```python
from build123d import *

# Parameters (mm, degrees)
SKETCH_1_R      = 1.5
SKETCH_1_R_2    = 2.1
EXTRUDE_1_DEPTH = 90
FILLET_1_R      = 1


with BuildPart() as part:
    # 草图1 → 凸台-拉伸1 (new, symmetric)
    with BuildSketch(Plane.XY):
        Polygon((-10, 10), (-10, 4.8), (-8.34, 3.14), (-8.34, 5.4), (-5.753553391, 5.4), (-3.8, 3.446446609), (-3.8, -3.446446609), (-5.753553391, -5.4), (-8.34, -5.4), (-8.34, -3.14), (-10, -4.8), (-10, -10), (-4.8, -10), (-3.14, -8.34), (-5.4, -8.34), (-5.4, -5.753553391), (-3.446446609, -3.8), (3.446446609, -3.8), (5.4, -5.753553391), (5.4, -8.34), (3.14, -8.34), (4.8, -10), (10, -10), (10, -4.8), (8.34, -3.14), (8.34, -5.4), (5.753553391, -5.4), (3.8, -3.446446609), (3.8, 3.446446609), (5.753553391, 5.4), (8.34, 5.4), (8.34, 3.14), (10, 4.8), (10, 10), (4.8, 10), (3.14, 8.34), (5.4, 8.34), (5.4, 5.753553391), (3.446446609, 3.8), (-3.446446609, 3.8), (-5.4, 5.753553391), (-5.4, 8.34), (-3.14, 8.34), (-4.8, 10), align=None)
        with Locations(Location((-7.5, 7.5, 0), (0, 0, 180))):
            Circle(SKETCH_1_R, mode=Mode.SUBTRACT)
        with Locations(Location((0, 0, 0), (0, 0, 180))):
            Circle(SKETCH_1_R_2, mode=Mode.SUBTRACT)
        with Locations(Location((-7.5, -7.5, 0), (0, 0, 180))):
            Circle(SKETCH_1_R, mode=Mode.SUBTRACT)
        with Locations(Location((7.5, -7.5, 0), (0, 0, 180))):
            Circle(SKETCH_1_R, mode=Mode.SUBTRACT)
        with Locations(Location((7.5, 7.5, 0), (0, 0, 180))):
            Circle(SKETCH_1_R, mode=Mode.SUBTRACT)
    extrude(amount=EXTRUDE_1_DEPTH, both=True)

    # 圆角1
    fillet_1_edges = [part.edges().sort_by_distance(p)[0] for p in [
        (10, 10, 0),
        (10, -10, 0),
        (-10, -10, 0),
        (-10, 10, 0),
    ]]
    fillet(fillet_1_edges, radius=FILLET_1_R)


solid = part.part
```
Here's how the part is built. I have some questions about the finished solid (model axes, mm). Round coordinates to 2 decimals unless told otherwise and drop trailing zeros. Order: outer loops, then holes, each group sorted by start corner. A loop starts at its lowest first (then second) coordinate and runs counter-clockwise, first axis right, second up. Notation, with made-up numbers: (-38.75, -24) -> (7.25, -24) arc R35 ccw to (7.25, 12) -> close; hole circle Ø5 at (45, 40.5). An arc over 180 degrees is marked (long way). Use a Markdown table: item, result. Add a question column.
(1) If we mould it in two halves opening along X, with no side actions, what happens to faces 1 (the face through (-10, -7, 1)), 2 (the face through (-7, -10, 1)), 3 (the face through (0, 3.8, 1)), 4 (the face through (8.7, -6.6, -1.3))? For each: released by +X, released by -X, zero draft, split by the parting line, or undercut.
(2) Suppose I cut it at A-A, the plane y = 0. Please give me the cut outline in (x, z).
(3) For pin 1 Ø5.5 at (y, z) = (0.5, 34) entering from +X; pin 2 Ø1.1 at (x, z) = (4, -30) entering from +Y; pin 3 Ø3 at (y, z) = (1, -57.5) entering from -X, each with a flat end and sliding along its axis, tell me the tip position at first contact or that it passes through.
(4) Suppose I cut it at C-C, the plane z = 49. Count the separate pieces of the cut face and the enclosed holes in it, and give its area (3 significant figures).
(5) I need wall thicknesses on line 1 along Y through (x, z) = (7.5, -14.5); line 2 along Y through (x, z) = (0, 4.5). Which ranges of each line are inside material? Lowest first, please.
Verdict:
| question | item | result |
|---|---|---|
| 1 | face 1 | released by -X |
| 1 | face 2 | zero draft |
| 1 | face 3 | undercut |
| 1 | face 4 | undercut |
| 2 | outline | (-3.8, -90) -> (-2.1, -90) -> (-2.1, 90) -> (-3.8, 90) -> close; (2.1, -90) -> (3.8, -90) -> (3.8, 90) -> (2.1, 90) -> close |
| 3 | pin 1 | x = 8.45 |
| 3 | pin 2 | y = 9.75 |
| 3 | pin 3 | x = -3.8 |
| 4 | separate pieces | 1 |
| 4 | enclosed holes | 5 |
| 4 | area | 123 mm2 |
| 5 | line 1 | -10 to -9, -6 to -5.4, 5.4 to 6, 9 to 10 |
| 5 | line 2 | -3.8 to -2.1, 2.1 to 3.8 |
